Input: part model. Units: mm. Frame: model coordinates. Face numbers are marked on the shaded views. A direction names the side the tool comes from. Give positions to 0.01 mm unless a question says otherwise; leave off trailing zeros. Loops run counter-clockwise (first coordinate to the right, second up) from the corner with the lowest first, then second, coordinate; pieces in that order, holes last. Notation, with made-up numbers: (-39.75, -23.5) -> (-21.75, -23.5) arc R5 cw to (-21.75, -15.5) -> close; hole circle Ø10 at (-37, 87.25). An arc over 180 degrees is marked (long way). Answer as a JSON object with one key per item and string values. Group by question number.
Autodesk Inventor part; units mm, degrees
ref_plane "YZ Plane" through (0, 0, 0) normal (1, 0, 0) x (0, 1, 0)
ref_plane "XZ Plane" through (0, 0, 0) normal (0, 1, 0) x (-1, 0, 0)
ref_plane "XY Plane" through (0, 0, 0) normal (0, 0, 1) x (1, 0, 0)
sketch "Schizzo1" plane through (0, 0, 0) normal (0, 1, 0) x (-1, 0, 0)
  line L0 (0, 0) -> (71, 0)
  line L1 (71, 0) -> (71, -64)
  line L2 (71, -64) -> (0, -64)
  line L3 (0, -64) -> (0, 0)
  dimension "d0" = 71
  dimension "d1" = 64
extrude "Estrusione1" add sketch "Schizzo1" along normal blind 29
shell "Svuotamento1" thickness 2 removed faces 1 at (-23.6667, 29, -21.3333)
fillet "Raccordo1" radius 2 4 edges at (0, 0, -32) (-35.5, 0, -64) (-35.5, 0, 0) (-71, 0, -32)
fillet "Raccordo2" radius 2 8 edges at (-0.5858, 0.5858, -63.4142) (0, 15.5, -64) (-0.5858, 0.5858, -0.5858) (0, 15.5, 0) (-70.4142, 0.5858, -63.4142) (-71, 15.5, -64) (-70.4142, 0.5858, -0.5858) (-71, 15.5, 0)
sketch "Schizzo3" plane through (-71, 2, -2) normal (-1, 0, 0) x (0, 0, 1)
  line L0 (-52.5, 27) -> (-27.5, 27)
  line L1 (-27.5, 27) -> (-27.5, 15)
  line L2 (-27.5, 15) -> (-52.5, 15)
  line L3 (-52.5, 15) -> (-52.5, 27)
  line L4 (-62, 27) -> (-62, 0)
  line L5 (-60, 27) -> (0, 27)
  line L6 (-60, 0) -> (-60, 27)
  line L7 (-60, 0) -> (-60, 27)
  point P0 (2, -2)
  dimension "d16" = 0
  dimension "d17" = 12
  dimension "d23" = 7.5
  dimension "d24" = 25
extrude "Estrusione3" cut sketch "Schizzo3" against normal up to next
chamfer "Smusso2" distance 2 angle 45 4 edges at (-70, 29, -54.5) (-70, 29, -29.5) (-70, 17, -29.5) (-70, 17, -54.5)
properties part number "Board_cover"
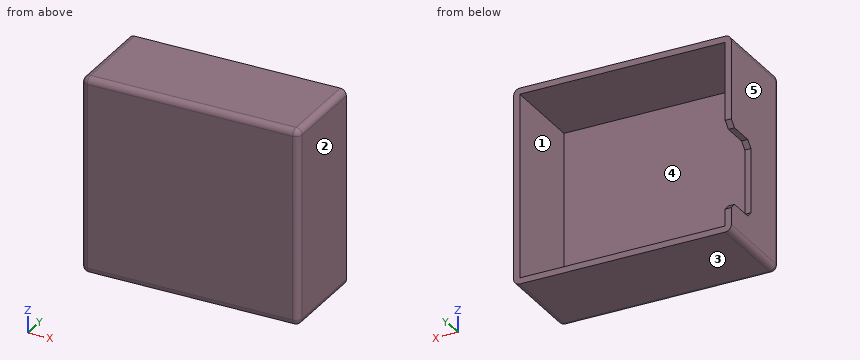
Q1. Pull-direction query (Z, two-part tool) for the marked faces 1, 2 and 3; classes: +Z half, -Z half, draft (parallel to the pull), parting line (faces both ways), or undercut.
Q2. Ray query, probe 1 along X at (y, z) = (4.5, -59.5); probe 2 along Z at (x, y) = (-44, 23.5); probe 3 along Y at (x, z) = (-23.5, -17.5). Return the intervals inside material, ascending.
Q3. Section A-A on y = 9. Return the cut outline in (x, z), then the cut area to 3 significant figures.
Q4. Section D-D on y = 26. Return the cut outline in (x, z).
Q5. Section B-B on z = -39. Return the cut outline in (x, y), then the cut area to 3 significant figures.
Q6. Section C-C on x = -60.5. Return the cut outline in (y, z).
Q7. Pin query (flat end, axial travel): pin 1 Ø1 at (x, z) = (-70, -43.5) entering from +Y; pin 2 Ø2 at (x, y) = (-70.5, 22) entering from -Z; pin 3 Ø0.6 at (x, y) = (-70, 23) entering from +Z. Return the tip coordinate at first contact, or that it passes through.
Q8. Set-up query: the marked faces 4 and 5. Return all of +Z, -Z, +X, -X, +Y, -Y with unobstructed straight access to the full face (end or side cutting, diameter ignored); none if empty.
Numbers:
{
 "1": {"face 1": "undercut", "face 2": "draft", "face 3": "-Z half"},
 "2": {"probe 1": "x = -71 to -69, -2 to 0", "probe 2": "z = -64 to -62, -2 to 0", "probe 3": "y = 0 to 2"},
 "3": {"outline": "(-71, -62) arc R2 ccw to (-69, -64) -> (-2, -64) arc R2 ccw to (0, -62) -> (0, -2) arc R2 ccw to (-2, 0) -> (-69, 0) arc R2 ccw to (-71, -2) -> close; hole (-69, -62) -> (-2, -62) -> (-2, -2) -> (-69, -2) -> close", "area": "521 mm²"},
 "4": {"outline": "(-71, -62) arc R2 ccw to (-69, -64) -> (-2, -64) arc R2 ccw to (0, -62) -> (0, -2) arc R2 ccw to (-2, 0) -> (-69, 0) arc R2 ccw to (-71, -2) -> (-71, -29.5) -> (-69, -29.5) -> (-69, -2) -> (-2, -2) -> (-2, -62) -> (-69, -62) -> (-69, -54.5) -> (-71, -54.5) -> close"},
 "5": {"outline": "(-71, 2) arc R2 ccw to (-69, 0) -> (-2, 0) arc R2 ccw to (0, 2) -> (0, 29) -> (-2, 29) -> (-2, 2) -> (-69, 2) -> (-69, 17) -> (-71, 17) -> close", "area": "224 mm²"},
 "6": {"outline": "(0, -62) arc R2 ccw to (2, -64) -> (29, -64) -> (29, -62) -> (2, -62) -> (2, -2) -> (29, -2) -> (29, 0) -> (2, 0) arc R2 ccw to (0, -2) -> close"},
 "7": {"pin 1": "stops at y = 17", "pin 2": "stops at z = -63.94", "pin 3": "stops at z = -0.13"},
 "8": {"face 4": "+Y", "face 5": "+Z, -Z, -X, +Y, -Y"}
}
